Here's the drawing with two shaded views (mm, measured from the low corner). I have some questions. A direction names the side the tool comes from. Give positions to 0.01 mm unless a question says otherwise; leave off trailing zeros. Order: outer loops, then holes, each group sorted by start corner. A loop starts at its lowest first (then second) coordinate and runs counter-clockwise, first axis right, second up. Notation, with made-up numbers: (36.25, 84.25) - (69.25, 84.25) arc R7 cw to (69.25, 92.25) - close; hole circle Ø7 at (21.25, 60.25). An arc over 180 degrees is marked (long way). Use one line per item in the form item = value. Start each with the question number.
1) Which directions (+Z, -Z, +X, -X, +Y, -Y) give clear straight access to the entire face, cutting with the end or side of a thin tool? Please do the marked faces 4 and 5.
2) Suppose I cut it at C-C, the plane x = 10.75. Write out the boundary of the cut face in (y, z), and give its area (3 significant figures).
3) Suppose I cut it at D-D, the plane z = 1.5. Write out the boundary of the cut face in (x, y).
4) Suppose I cut it at B-B, the plane y = 15. Write out the boundary of the cut face in (x, z).
5) Please list where these lines run through material, in increasing order: probe 1 along X at (y, z) = (24.5, 3.25); probe 2 along Y at (x, z) = (2.3, 7.5); probe 3 along Z at (x, y) = (13, 53.25).
6) For pin 1 (1 mm diameter, centred on x = 15, z = 12, fed in from -Y); pin 2 (5 mm diameter, centred on y = 7.5, z = 7.5, fed in from -X), each with a flat end and sliding along its axis, tell me the tip position at first contact or that it passes through.
7) Suppose I cut it at A-A, the plane z = 7.5. Write out the boundary of the cut face in (x, y).
8) We'd pull the mould along X, two halves only. Please class the marked faces 1, 2 and 3: released by +X, released by -X, zero draft, split by the parting line, or undercut.
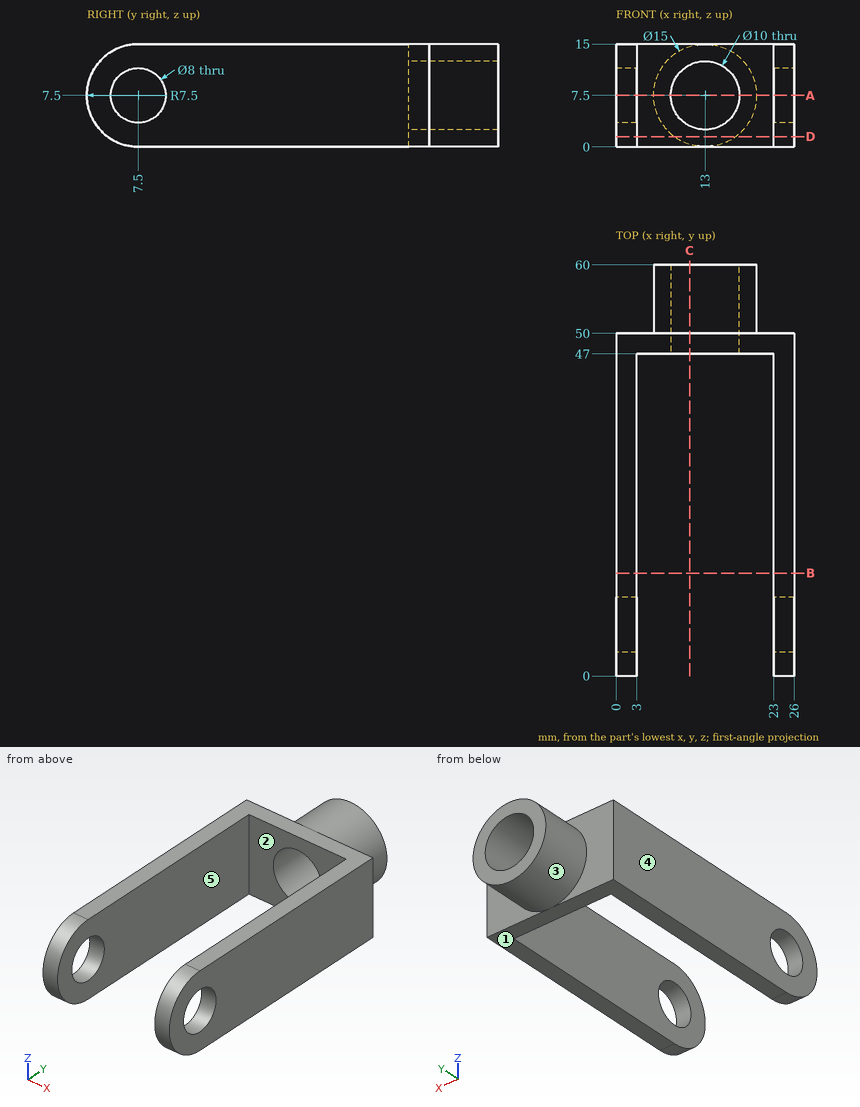
Result sheet:
q1.face_4 = +Z, -Z, -X, +Y, -Y
q1.face_5 = +Z, -Z, -Y
q2.outline = (47, 0) - (50, 0) - (50, 0.35) - (60, 0.35) - (60, 3.03) - (47, 3.03) - close; (47, 11.97) - (60, 11.97) - (60, 14.65) - (50, 14.65) - (50, 15) - (47, 15) - close
q2.area = 72.0 mm²
q3.outline = (0, 3) - (3, 3) - (3, 47) - (23, 47) - (23, 3) - (26, 3) - (26, 50) - (17.5, 50) - (17.5, 60) - (8.5, 60) - (8.5, 50) - (0, 50) - close
q4.outline = (0, 0) - (3, 0) - (3, 15) - (0, 15) - close; (23, 0) - (26, 0) - (26, 15) - (23, 15) - close
q5.probe_1 = 0 to 3, 23 to 26
q5.probe_2 = 0 to 3.5, 11.5 to 50
q5.probe_3 = 0 to 2.5, 12.5 to 15
q6.pin_1 = 47
q6.pin_2 = through
q7.outline = (0, 0) - (3, 0) - (3, 3.5) - (0, 3.5) - close; (0, 11.5) - (3, 11.5) - (3, 47) - (8, 47) - (8, 60) - (5.5, 60) - (5.5, 50) - (0, 50) - close; (18, 47) - (23, 47) - (23, 11.5) - (26, 11.5) - (26, 50) - (20.5, 50) - (20.5, 60) - (18, 60) - close; (23, 0) - (26, 0) - (26, 3.5) - (23, 3.5) - close
q8.face_1 = zero draft
q8.face_2 = undercut
q8.face_3 = split by the parting line
